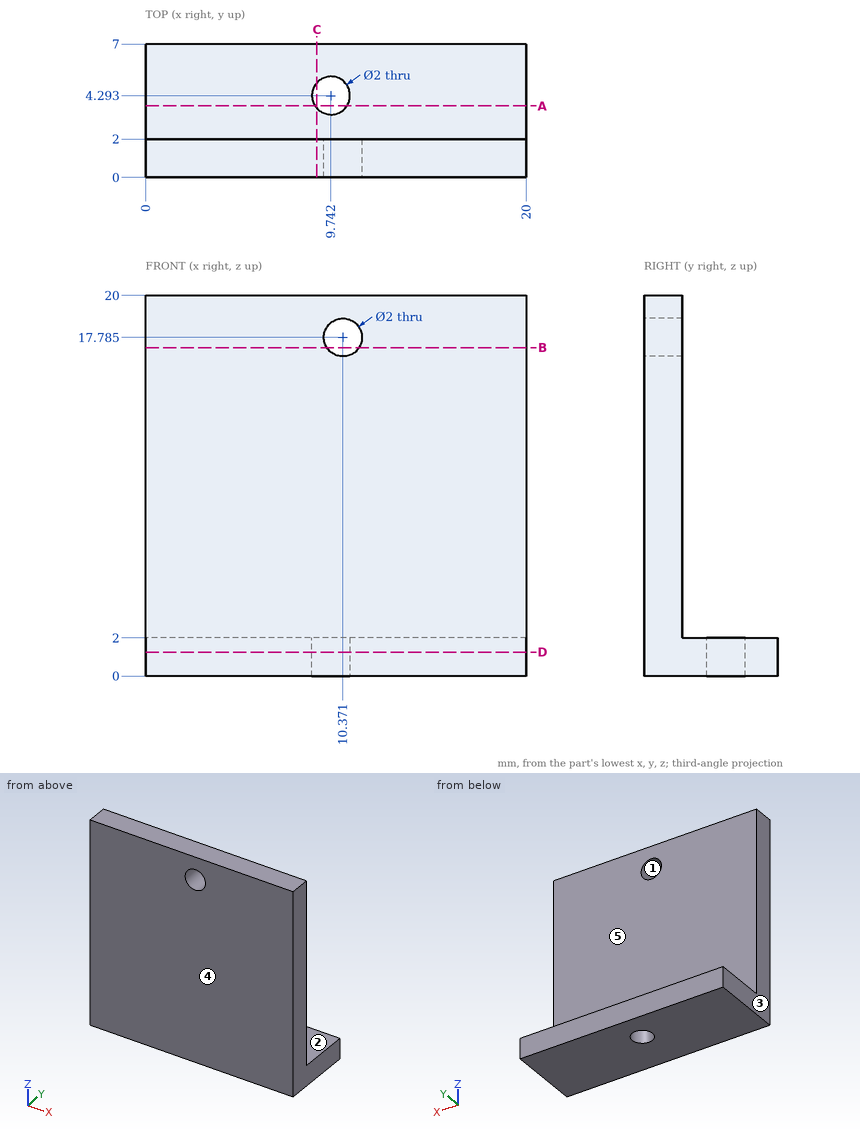
Study the drawing (mm; zero at the part's minimum x, y, z) and answer. A direction names the side the tool comes from. Round coordinates to 2 decimals unless told otherwise and drop trailing zeros. Order: outer loops, then holes, each group sorted by start corner. A loop starts at its lowest first (then second) coordinate and runs counter-clockwise, first axis right, second up. Notation, with made-up numbers: (52.5, 81) -> (106.5, 81) arc R30 cw to (106.5, 110) -> close; hole circle Ø2 at (-26.5, 79). An arc over 180 degrees is marked (long way). Write each question's results on one line, items separated by ' | '. Start each with the question number.
Q1. Find section C-C (x = 9). Determine the outline of the cut face in (y, z).
Q2. Find section D-D (z = 1.25). Determine the outline of the cut face in (x, y), then the cut area to 3 significant figures.
Q3. Each of these flat-tipped pins is pushed along its axis until it touches: pin 1 (2 mm diameter, centred on x = 18, y = 5.5, fed in from +Z); pin 2 (9 mm diameter, centred on x = 6, z = 15, fed in from +Y). Where does it stop, or does it pass through?
Q4. Find section B-B (z = 17.25). Determine the outline of the cut face in (x, y).
Q5. Which of the six approach directions +Z, -Z, +X, -X, +Y, -Y give full straight-line access (tool end or side, diameter ignored) to the marked faces 4 and 5?
Q6. A straight line is drawn through the part: probe 1 along Y at (x, z) = (17.25, 6.5). Find the intervals that lie inside material, in ascending order. Write a range as from..to.
Q7. The mould has two halves that part along X. Classify the marked faces 1, 2 and 3: pulls with the +X half, pulls with the -X half, needs draft (parallel to the pull), parting line crosses it, or undercut.
Q8. Find section A-A (y = 3.75). Determine the outline of the cut face in (x, z).
Worked answers:
1) outline: (0, 0) -> (3.62, 0) -> (3.62, 2) -> (2, 2) -> (2, 20) -> (0, 20) -> close; (4.96, 0) -> (7, 0) -> (7, 2) -> (4.96, 2) -> close
2) outline: (0, 0) -> (20, 0) -> (20, 7) -> (0, 7) -> close; hole circle Ø2 at (9.74, 4.29) | area: 137 mm2
3) pin 1: stops at z = 2 | pin 2: stops at y = 2
4) outline: (0, 0) -> (9.53, 0) -> (9.53, 2) -> (0, 2) -> close; (11.22, 0) -> (20, 0) -> (20, 2) -> (11.22, 2) -> close
5) face 4: +Z, -Z, +X, -X, -Y | face 5: +Z, +X, -X, +Y
6) probe 1: y = 0..2
7) face 1: undercut | face 2: needs draft | face 3: pulls with the -X half
8) outline: (0, 0) -> (8.9, 0) -> (8.9, 2) -> (0, 2) -> close; (10.58, 0) -> (20, 0) -> (20, 2) -> (10.58, 2) -> close
